Read the model definition and answer for the solid it produces. Units are mm, in the model's axes. A direction names the side the tool comes from. Coordinates: 2 decimals unless noted, no trailing zeros. Write each loop counter-clockwise with the first axis right and the second up, starting at its lowest first coordinate (ties: lowest second). Pieces come first, ordered by that corner, then holes.
Item 1: Section B-B (y = 5.3) is taken. Give the vertices of the cut face in (x, z).
Item 2: Section D-D (z = 4) is taken. Give the vertices of the cut face in (x, y).
Item 3: Section A-A (z = -4) is taken. Give the vertices of the cut face in (x, y), then the cut area to 3 significant figures.
Item 4: A tool of negligible diameter and unlimited length cuts with its end or side. For faces 4 (the face through (48.05, 5.35, 0.51)), 5 (the face through (4, 4, -5)), 6 (the face through (27, 19, 1)), from which of +Z, -Z, +X, -X, +Y, -Y can it reach the whole face along a straight path? Write none if from no direction.
Item 5: Straight lines are drawn through the part: probe 1 along Y at (x, z) = (26.7, 5.45); probe 2 along X at (y, z) = (40, 3.75); probe 3 along Y at (x, z) = (44, -6). For each, find the intervals that lie inside material, in ascending order.
Item 6: Each of these flat-tipped pins is pushed along its axis until it touches: P1, Ø1.5, axis at x = 22, z = 1.5, coming from the -Y side; P2, Ø4, axis at x = 14.5, y = 40, coming from the -Z side. Where does it stop, or does it pass through?
Item 7: Determine the mould class of faces 1 (the face through (15.9, 21, -5)), 2 (the face through (0.57, 103.7, -1.69)), 3 (the face through (53.73, 0.6, -4.37)) for opening direction Y: released by +Y, released by -Y, zero draft, split by the parting line, or undercut.
Item 8: Section C-C (y = 64) is taken. Give the vertices of the cut face in (x, z), then the cut area to 3 significant figures.
from build123d import *

# Parameters (mm, degrees)
SKICA1_W                 = 54.3
SKICA1_H                 = 36.5
P_IDAT_VYSUNUT_M1_DEPTH  = 1
SKICA4_W                 = 54.3
SKICA4_H                 = 67.8
SKICA4_W_2               = 51
SKICA4_H_2               = 64.5
P_IDAT_VYSUNUT_M2_DEPTH  = 6
SKICA5_W                 = 51
SKICA5_H                 = 64.5
P_IDAT_VYSUNUT_M3_DEPTH  = 1
SKICA2_R                 = 1.1
ODEBRAT_VYSUNUT_M1_DEPTH = 1
SKICA3_R                 = 5.25
SKICA3_R_2               = 2.75
SKICA3_W                 = 17
SKICA3_H                 = 3.5
ODEBRAT_VYSUNUT_M2_DEPTH = 1
SKICA6_W                 = 41
SKICA6_H                 = 38
SKICA6_R                 = 2.25
SKICA6_R_2               = 1.1
SKICA6_W_2               = 13
SKICA6_H_2               = 10
ODEBRAT_VYSUNUT_M3_DEPTH = 118.74115678
SKICA8_W                 = 54.3
SKICA8_H                 = 104.3
SKICA8_W_2               = 51
SKICA8_H_2               = 101
P_IDAT_VYSUNUT_M4_DEPTH  = 9.6
ZAOBLIT1_R               = 2
SKICA9_W                 = 5
SKICA9_H                 = 5
P_IDAT_VYSUNUT_M5_DEPTH  = 9.6


with BuildPart() as part:
    # Skica1 → Přidat vysunutím1 (new body)
    with BuildSketch(Plane.XY):
        with Locations((27.15, 18.25)):
            Rectangle(SKICA1_W, SKICA1_H)
    extrude(amount=P_IDAT_VYSUNUT_M1_DEPTH)

    # Skica4 → Přidat vysunutím2 (add)
    with BuildSketch(Plane.XY):
        with Locations((27.15, 70.4)):
            Rectangle(SKICA4_W, SKICA4_H)
        with Locations((27.15, 70.4)):
            Rectangle(SKICA4_W_2, SKICA4_H_2, mode=Mode.SUBTRACT)
    extrude(amount=P_IDAT_VYSUNUT_M2_DEPTH)

    # Skica5 → Přidat vysunutím3 (add)
    with BuildSketch(Plane.XY.offset(6)):
        with Locations((27.15, 70.4)):
            Rectangle(SKICA5_W, SKICA5_H)
    extrude(amount=-P_IDAT_VYSUNUT_M3_DEPTH)

    # Skica2 → Odebrat vysunutím1 (cut)
    with BuildSketch(Plane.XY.offset(1)):
        with Locations((49.15, 5.3)):
            Circle(SKICA2_R)
        with Locations((5.15, 5.3)):
            Circle(SKICA2_R)
    extrude(amount=-ODEBRAT_VYSUNUT_M1_DEPTH, mode=Mode.SUBTRACT)

    # Skica3 → Odebrat vysunutím2 (cut)
    with BuildSketch(Plane.XY.offset(1)):
        with Locations((9.15, 11.5)):
            Circle(SKICA3_R)
        with Locations((21.15, 11.5)):
            Circle(SKICA3_R)
        with Locations((33.15, 11.5)):
            Circle(SKICA3_R)
        with Locations((45.15, 11.5)):
            Circle(SKICA3_R)
        with Locations((7.2, 32.6)):
            Circle(SKICA3_R_2)
        with Locations((31.55, 32.75)):
            Rectangle(SKICA3_W, SKICA3_H)
    extrude(amount=-ODEBRAT_VYSUNUT_M2_DEPTH, mode=Mode.SUBTRACT)

    # Skica6 → Odebrat vysunutím3 (cut, through all)
    with BuildSketch(Plane.XY.offset(6)):
        with Locations((24.8, 78)):
            Rectangle(SKICA6_W, SKICA6_H)
        with Locations((34.7, 47)):
            Circle(SKICA6_R)
        with Locations((26.7, 47)):
            Circle(SKICA6_R)
        with Locations((18.7, 47)):
            Circle(SKICA6_R)
        with Locations((10.7, 47)):
            Circle(SKICA6_R)
        with Locations((5.15, 99.2)):
            Circle(SKICA6_R_2)
        with Locations((45.8, 46.8)):
            Rectangle(SKICA6_W_2, SKICA6_H_2)
    extrude(amount=-ODEBRAT_VYSUNUT_M3_DEPTH, mode=Mode.SUBTRACT)

    # Skica8 → Přidat vysunutím4 (add)
    with BuildSketch(Plane(origin=(0, 0, 0), x_dir=(-1, 0, 0), z_dir=(0, 0, -1))):
        with Locations((-27.15, 52.15)):
            Rectangle(SKICA8_W, SKICA8_H)
        with Locations((-27.15, 52.15)):
            Rectangle(SKICA8_W_2, SKICA8_H_2, mode=Mode.SUBTRACT)
    extrude(amount=P_IDAT_VYSUNUT_M4_DEPTH)

    # Zaoblit1
    zaoblit1_edges = [part.edges().sort_by_distance(p)[0] for p in [
        (0, 104.3, -1.8),
        (54.3, 104.3, -1.8),
        (54.3, 0, -4.3),
        (0, 0, -4.3),
    ]]
    fillet(zaoblit1_edges, radius=ZAOBLIT1_R)

    # Skica9 → Přidat vysunutím5 (add)
    with BuildSketch(Plane(origin=(0, 0, 0), x_dir=(-1, 0, 0), z_dir=(0, 0, -1))):
        Polygon((-1.65, 1.65), (-1.65, 6.35), (-6.35, 1.65), align=None)
        Polygon((-52.65, 1.65), (-52.65, 6.35), (-47.95, 1.65), align=None)
        with Locations((-18.4, 21.25)):
            Rectangle(SKICA9_W, SKICA9_H)
    extrude(amount=P_IDAT_VYSUNUT_M5_DEPTH)


solid = part.part
Established:
1. outline: (0, -9.6) - (2.7, -9.6) - (2.7, 0) - (4.05, 0) - (4.05, 1) - (0, 1) - close; (6.25, 0) - (48.05, 0) - (48.05, 1) - (6.25, 1) - close; (50.25, 0) - (51.6, 0) - (51.6, -9.6) - (54.3, -9.6) - (54.3, 1) - (50.25, 1) - close
2. outline: (0, 36.5) - (54.3, 36.5) - (54.3, 102.3) arc R2 ccw to (52.3, 104.3) - (2, 104.3) arc R2 ccw to (0, 102.3) - close; hole (1.65, 38.15) - (52.65, 38.15) - (52.65, 102.65) - (1.65, 102.65) - close
3. outline: (0, 2) arc R2 ccw to (2, 0) - (52.3, 0) arc R2 ccw to (54.3, 2) - (54.3, 102.3) arc R2 ccw to (52.3, 104.3) - (2, 104.3) arc R2 ccw to (0, 102.3) - close; (15.9, 18.75) - (20.9, 18.75) - (20.9, 23.75) - (15.9, 23.75) - close; hole (1.65, 6.35) - (6.35, 1.65) - (47.95, 1.65) - (52.65, 6.35) - (52.65, 102.65) - (1.65, 102.65) - close
3. area: 556 mm2
4. face 4: +Z, -Z
4. face 5: -Z
4. face 6: +Z, +X, -X, -Y
5. probe 1: y = 36.5 to 44.75, 49.25 to 59, 97 to 104.3
5. probe 2: x = 0 to 1.65, 52.65 to 54.3
5. probe 3: y = 0 to 1.65, 102.65 to 104.3
6. P1: stops at y = 0
6. P2: stops at z = 0
7. face 1: undercut
7. face 2: released by +Y
7. face 3: released by -Y
8. outline: (0, -9.6) - (1.65, -9.6) - (1.65, 5) - (4.3, 5) - (4.3, 6) - (0, 6) - close; (45.3, 5) - (52.65, 5) - (52.65, -9.6) - (54.3, -9.6) - (54.3, 6) - (45.3, 6) - close
8. area: 61.5 mm2
